from build123d import *

# Parameters (mm, degrees)
SKETCH_1_W      = 40
SKETCH_1_H      = 70
EXTRUDE_1_DEPTH = 2
SKETCH_2_W      = 40
SKETCH_2_H      = 2
EXTRUDE_2_DEPTH = 22


with BuildPart() as part:
    # 草图1 → 凸台-拉伸1 (new body)
    with BuildSketch(Plane.XY):
        with Locations((-10.271445819, -4.719420773)):
            Rectangle(SKETCH_1_W, SKETCH_1_H)
        with BuildLine():
            Line((-25.271445819, -1.469420773), (-21.271445819, -1.469420773))
            Line((-21.271445819, -1.469420773), (-17.171194561, -1.469420773))
            ThreePointArc((-17.171194561, -1.469420773), (-12.103842793, 13.946987092), (2.728554181, 20.530579227))
            Line((2.728554181, 20.530579227), (2.728554181, 25.730579227))
            ThreePointArc((2.728554181, 25.730579227), (-14.368814038, 19.043277572), (-22.391955368, 2.530579227))
            Line((-22.391955368, 2.530579227), (-25.271445819, 2.530579227))
            ThreePointArc((-25.271445819, 2.530579227), (-27.271445819, 0.530579227), (-25.271445819, -1.469420773))
        make_face(mode=Mode.SUBTRACT)
    extrude(amount=EXTRUDE_1_DEPTH)

    # 草图2 → 凸台-拉伸2 (add)
    with BuildSketch(Plane.XY.offset(2)):
        with Locations((-10.271445819, -38.719420773)):
            Rectangle(SKETCH_2_W, SKETCH_2_H)
    extrude(amount=-EXTRUDE_2_DEPTH)


solid = part.part
CAD build for the part. Positions are in the model's coordinates, mm. A direction names the side the tool comes from. Coordinates: 2 decimals unless noted, no trailing zeros. Write each loop counter-clockwise with the first axis right and the second up, starting at its lowest first coordinate (ties: lowest second). Pieces come first, ordered by that corner, then holes. Notation, with made-up numbers: M 52,-11.5 L 96,-11.5 A16 ccw 96,15.5 Z; hole C 8,63 d8. An arc over 180 degrees is marked long. Return JSON: item names as keys, results as strings.
Item 1: Slice it at D-D, the plane x = -14.5. Write the cut outline in (y, z).
Findings below:
{"outline": "M -39.72,-20 L -37.72,-20 L -37.72,0 L 10.69,0 L 10.69,2 L -39.72,2 Z; M 18.92,0 L 30.28,0 L 30.28,2 L 18.92,2 Z"}
Item 2: Which spindle directions (+Z, -Z, +X, -X, +Y, -Y) get a long thin tool onto all of the face, cutting with end or side? Do faces 4 (the flat face through (-11, -3, 0)), 5 (the cylindrical face through (-27.27, 0.57, 0.99)), 6 (the flat face through (-11, -39, -20)). Say none if no direction does.
Findings below:
{"face 4": "-Z, +X, -X, +Y", "face 5": "+Z, -Z", "face 6": "-Z, +X, -X, +Y, -Y"}
Item 3: Probe line 1 (Z direction, x = 6, y = 10); line 2 (Y direction, x = -15.5, z = -5); line 3 (Y direction, x = -9, z = 1). List the from-to ranges inside material, lowest first. Write a range as from..to.
Findings below:
{"line 1": "z = 0..2", "line 2": "y = -39.72..-37.72", "line 3": "y = -39.72..16.73, 22.83..30.28"}
Item 4: Slice it at A-A, the plane y = 16.5. Write the cut outline in (x, z), and give its area (3 significant figures).
Findings below:
{"outline": "M -30.27,0 L -16.77,0 L -16.77,2 L -30.27,2 Z; M -9.31,0 L 9.73,0 L 9.73,2 L -9.31,2 Z", "area": "65.1 mm2"}
Item 5: Slice it at C-C, the plane z = -10. Write the cut outline in (x, y), and give its area (3 significant figures).
Findings below:
{"outline": "M -30.27,-39.72 L 9.73,-39.72 L 9.73,-37.72 L -30.27,-37.72 Z", "area": "80.0 mm2"}
Item 6: Two-plate mould, pull along Y, no slides. Class faces 1 (the flat face through (-11, -4, 2)), 2 (the flat face through (-11, -37.719, -10)), 3 (the cylindrical face through (-14.2, 19.2, 1)): +Y half, -Y half, draft (parallel to the pull), parting line (faces both ways), or undercut.
Findings below:
{"face 1": "draft", "face 2": "+Y half", "face 3": "undercut"}
Item 7: Drop flat-ended pins along their axis: pin 1 Ø3 at (x, z) = (-2, -17.5) entering from +Y; pin 2 Ø12 at (x, y) = (-26, 20.5) entering from -Z. Give the stop position or say it passes through.
Findings below:
{"pin 1": "stops at y = -37.72", "pin 2": "stops at z = 0"}
Item 8: Slice it at B-B, the plane x = -7.5. Write the cut outline in (y, z).
Findings below:
{"outline": "M -39.72,-20 L -37.72,-20 L -37.72,0 L 17.72,0 L 17.72,2 L -39.72,2 Z; M 23.56,0 L 30.28,0 L 30.28,2 L 23.56,2 Z"}
